Check sheet for the modelled part. Datum: model origin and axes. Units: mm. Face numbers are marked on the shaded views. A direction names the side the tool comes from. Round coordinates to 2 decimals unless told otherwise and drop trailing zeros. Order: outer loops, then holes, each group sorted by start corner. A loop starts at its lowest first (then second) coordinate and runs counter-clockwise, first axis right, second up.
(1) Thickness scan on probe 1 along Y at (x, z) = (-3.1, 6.75); probe 2 along X at (y, z) = (1, 4.5); probe 3 along X at (y, z) = (-0.25, 33.5). Record the ranges inside material, lowest first.
(2) Sectioned sample at B-B, the plane z = 5. Count the separate pieces of the cut face and the enclosed holes in it, and give its area (3 significant figures).
(3) Depth check by flat-ended pin: pin 1 (6 mm diameter, centred on y = 6.5, z = 20.5, fed in from -X); pin 2 (0.8 mm diameter, centred on y = 9, z = 19.5, fed in from -X); pin 3 (6 mm diameter, centred on x = -2.5, z = 8.5, fed in from -Y). Enter the tip coordinate at first touch or a pass-through.
(4) Mould release check, pull along Y, two halves, no side actions. Record for the marked faces 4, 5, 6 and 7: released by +Y, released by -Y, zero draft, split by the parting line, or undercut.
(5) Sectioned sample at D-D, the plane y = -3.1. Enter the section's corners in (x, z).
(6) Tool access check on the marked faces 1, 2 and 3. Record the directions out of +Z, -Z, +X, -X, +Y, -Y that give a thin tool (end or side, any length) a straight path to the whole face; none if there is none.
(7) Sectioned sample at A-A, the plane y = -12. Enter the section's corners in (x, z), and give its area (3 significant figures).
(8) Sectioned sample at C-C, the plane z = 27.5. Enter the section's corners in (x, y), and give its area (3 significant figures).
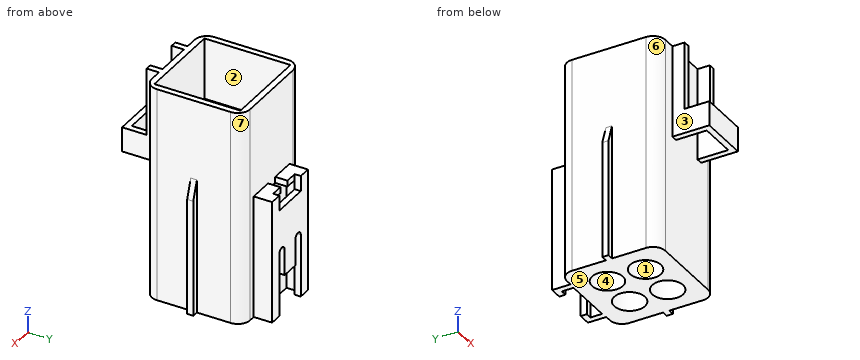
```python
from build123d import *

# Parameters (mm, degrees)
SKETCH_1_W           = 16
SKETCH_1_H           = 16
EXTRUDE_1_DEPTH      = 35
FILLET_1_R           = 2
SKETCH_2_W           = 8
SKETCH_2_H           = 15
EXTRUDE_2_DEPTH      = 6
CUT_EXTRUDE_2_REACH  = 40.536
SKETCH_3_W           = 6
SKETCH_3_H           = 5
SKETCH_7_W           = 8
SKETCH_7_H           = 4
CUT_EXTRUDE_4_DEPTH  = 11
SKETCH_8_W           = 10
SKETCH_8_H           = 20
EXTRUDE_3_DEPTH      = 3
SKETCH_9_W           = 6
SKETCH_9_H           = 2.5
CUT_EXTRUDE_5_DEPTH  = 1
FILLET_2_R           = 0.75
SKETCH_10_R          = 2.5
CUT_EXTRUDE_6_DEPTH  = 10
SKETCH_11_W          = 14
SKETCH_11_H          = 14
CUT_EXTRUDE_7_DEPTH  = 10
SKETCH_12_W          = 8
SKETCH_12_H          = 1.908274713
CUT_EXTRUDE_8_DEPTH  = 19
SKETCH_13_W          = 2
SKETCH_13_H          = 1
CUT_EXTRUDE_9_DEPTH  = 2
SKETCH_14_W          = 22
SKETCH_14_H          = 1
EXTRUDE_4_DEPTH      = 1
CUT_EXTRUDE_10_DEPTH = 1


with BuildPart() as part:
    # ｽｹｯﾁ1 → ﾎﾞｽ - 押し出し1 (new body)
    with BuildSketch(Plane.XY):
        Rectangle(SKETCH_1_W, SKETCH_1_H)
    extrude(amount=EXTRUDE_1_DEPTH)

    # ﾌｨﾚｯﾄ1
    fillet_1_edges = [part.edges().sort_by_distance(p)[0] for p in [
        (-8, 8, 17.5),
        (8, 8, 17.5),
        (8, -8, 17.5),
        (-8, -8, 17.5),
    ]]
    fillet(fillet_1_edges, radius=FILLET_1_R)

    # ｽｹｯﾁ2 → ﾎﾞｽ - 押し出し2 (add)
    with BuildSketch(Plane.XZ.offset(8)):
        with Locations((0, 27.5)):
            Rectangle(SKETCH_2_W, SKETCH_2_H)
    extrude(amount=EXTRUDE_2_DEPTH)

    # ｽｹｯﾁ3 → ｶｯﾄ - 押し出し2 (cut, up to next)
    with BuildSketch(Plane.XY.offset(35), mode=Mode.PRIVATE) as cut_extrude_2_sk1:
        with Locations((0, -10.5)):
            Rectangle(SKETCH_3_W, SKETCH_3_H)
    cut_extrude_2_tool1 = extrude(cut_extrude_2_sk1.sketch, amount=-CUT_EXTRUDE_2_REACH, mode=Mode.PRIVATE) & part.part
    add(cut_extrude_2_tool1.solids().sort_by_distance((0, -10.5, 35))[0], mode=Mode.SUBTRACT)

    # ｽｹｯﾁ7 → ｶｯﾄ - 押し出し4 (cut)
    with BuildSketch(Plane.XY.offset(35)):
        with Locations((0, -12)):
            Rectangle(SKETCH_7_W, SKETCH_7_H)
    extrude(amount=-CUT_EXTRUDE_4_DEPTH, mode=Mode.SUBTRACT)

    # ｽｹｯﾁ8 → ﾎﾞｽ - 押し出し3 (add)
    with BuildSketch(Plane(origin=(0, 8, 0), x_dir=(1, 0, 0), z_dir=(0, 1, 0))):
        with Locations((0, -10)):
            Rectangle(SKETCH_8_W, SKETCH_8_H)
    extrude(amount=EXTRUDE_3_DEPTH)

    # ｽｹｯﾁ9 → ｶｯﾄ - 押し出し5 (cut)
    with BuildSketch(Plane(origin=(0, 11, 0), x_dir=(1, 0, 0), z_dir=(0, 1, 0))):
        Polygon((3, 0), (3, -11), (1.5, -11), (1.5, -6), (-1.5, -6), (-1.5, -11), (-3, -11), (-3, 0), align=None)
        with Locations((0, -18.75)):
            Rectangle(SKETCH_9_W, SKETCH_9_H)
    extrude(amount=-CUT_EXTRUDE_5_DEPTH, mode=Mode.SUBTRACT)

    # ﾌｨﾚｯﾄ2
    fillet_2_edges = [part.edges().sort_by_distance(p)[0] for p in [
        (-3, 10.5, 11),
        (-1.5, 10.5, 11),
        (1.5, 10.5, 11),
        (3, 10.5, 11),
    ]]
    fillet(fillet_2_edges, radius=FILLET_2_R - 0.0001)  # a hair under: the kernel refuses the full size

    # ｽｹｯﾁ10 → ｶｯﾄ - 押し出し6 (cut)
    with BuildSketch(Plane(origin=(0, 0, 0), x_dir=(-1, 0, 0), z_dir=(0, 0, -1))):
        with Locations((-3.1, 3.1)):
            Circle(SKETCH_10_R)
        with Locations(Location((3.1, 3.1, 0), (0, 0, 180))):
            Circle(SKETCH_10_R)
        with Locations((3.1, -3.1)):
            Circle(SKETCH_10_R)
        with Locations(Location((-3.1, -3.1, 0), (0, 0, 180))):
            Circle(SKETCH_10_R)
    extrude(amount=-CUT_EXTRUDE_6_DEPTH, mode=Mode.SUBTRACT)

    # ｽｹｯﾁ11 → ｶｯﾄ - 押し出し7 (cut)
    with BuildSketch(Plane.XY.offset(35)):
        Rectangle(SKETCH_11_W, SKETCH_11_H)
    extrude(amount=-CUT_EXTRUDE_7_DEPTH, mode=Mode.SUBTRACT)

    # ｽｹｯﾁ12 → ｶｯﾄ - 押し出し8 (cut)
    with BuildSketch(Plane(origin=(0, 0, 0), x_dir=(-1, 0, 0), z_dir=(0, 0, -1))):
        with Locations((0, 9.045862644)):
            Rectangle(SKETCH_12_W, SKETCH_12_H)
    extrude(amount=-CUT_EXTRUDE_8_DEPTH, mode=Mode.SUBTRACT)

    # ｽｹｯﾁ13 → ｶｯﾄ - 押し出し9 (cut)
    with BuildSketch(Plane(origin=(0, 10, 0), x_dir=(1, 0, 0), z_dir=(0, 1, 0))):
        with Locations((0, -19.5)):
            Rectangle(SKETCH_13_W, SKETCH_13_H)
    extrude(amount=-CUT_EXTRUDE_9_DEPTH, mode=Mode.SUBTRACT)

    # ｽｹｯﾁ14 → ﾎﾞｽ - 押し出し4 (add)
    with BuildSketch(Plane(origin=(8, 0, 0), x_dir=(0, 0, -1), z_dir=(1, 0, 0))):
        with Locations((-11, 0)):
            Rectangle(SKETCH_14_W, SKETCH_14_H)
    extrude_4 = extrude(amount=EXTRUDE_4_DEPTH)

    # ｽｹｯﾁ16 → ｶｯﾄ - 押し出し10 (cut)
    with BuildSketch(Plane(origin=(0, 0.5, 0), x_dir=(1, 0, 0), z_dir=(0, 1, 0))):
        Polygon((8, -22), (9, -22), (9, -19), align=None)
    cut_extrude_10 = extrude(amount=-CUT_EXTRUDE_10_DEPTH, mode=Mode.SUBTRACT)

    # ﾐﾗｰ1: ﾎﾞｽ - 押し出し4 across plane
    add(extrude_4.mirror(Plane(origin=(0, 0, 0), x_dir=(0, 0, 1), z_dir=(1, 0, 0))))

    # ﾐﾗｰ2: ｶｯﾄ - 押し出し10 across plane
    add(cut_extrude_10.mirror(Plane(origin=(0, 0, 0), x_dir=(0, 0, 1), z_dir=(1, 0, 0))), mode=Mode.SUBTRACT)


solid = part.part
```
Derived:
1. probe 1: y = -8 to -5.6, -0.6 to 0.6, 5.6 to 8.09, 10 to 11
1. probe 2: x = -8 to -4.46, -1.74 to 1.74, 4.46 to 8
1. probe 3: x = -8 to -7, 7 to 8
2. separate pieces: 1
2. enclosed holes: 4
2. area: 185 mm2
3. pin 1: stops at x = -8
3. pin 2: stops at x = -5
3. pin 3: stops at y = -8
4. face 4: undercut
4. face 5: zero draft
4. face 6: released by -Y
4. face 7: released by +Y
5. outline: (-8, 0) - (-5.6, 0) - (-5.6, 10) - (-0.6, 10) - (-0.6, 0) - (0.6, 0) - (0.6, 10) - (5.6, 10) - (5.6, 0) - (8, 0) - (8, 35) - (7, 35) - (7, 25) - (-7, 25) - (-7, 35) - (-8, 35) - close
6. face 1: -Z
6. face 2: +Z
6. face 3: +Z, -Z, -X, -Y
7. outline: (-4, 20) - (-3, 20) - (-3, 24) - (-4, 24) - close; (3, 20) - (4, 20) - (4, 24) - (3, 24) - close
7. area: 8.00 mm2
8. outline: (-8, -6) arc R2 ccw to (-6, -8) - (-4, -8) - (-4, -10) - (-3, -10) - (-3, -8) - (3, -8) - (3, -10) - (4, -10) - (4, -8) - (6, -8) arc R2 ccw to (8, -6) - (8, 6) arc R2 ccw to (6, 8) - (-6, 8) arc R2 ccw to (-8, 6) - close; hole (-7, -7) - (7, -7) - (7, 7) - (-7, 7) - close
8. area: 60.6 mm2
